from build123d import *

# Parameters (mm, degrees)
SKETCH1_W           = 200
SKETCH1_H           = 30
SKETCH1_W_2         = 20
SKETCH1_H_2         = 200
SKETCH1_R           = 4
BOSS_EXTRUDE1_DEPTH = 1


with BuildPart() as part:
    # Sketch1 → Boss-Extrude1 (new body)
    with BuildSketch(Plane.XY):
        with Locations((120, 100)):
            Rectangle(SKETCH1_W, SKETCH1_H)
        with Locations((10, 100)):
            Rectangle(SKETCH1_W_2, SKETCH1_H_2)
        with Locations((10, 175)):
            Circle(SKETCH1_R, mode=Mode.SUBTRACT)
        with Locations((10, 25)):
            Circle(SKETCH1_R, mode=Mode.SUBTRACT)
        Polygon((220, 200), (220, 115), (220, 85), (220, 0), (240, 0), (240, 200), align=None)
        with Locations((230, 25)):
            Circle(SKETCH1_R, mode=Mode.SUBTRACT)
        with Locations((230, 175)):
            Circle(SKETCH1_R, mode=Mode.SUBTRACT)
    extrude(amount=BOSS_EXTRUDE1_DEPTH)


solid = part.part
For this review, take the finished solid that the model builds, in its own axes (mm). Give positions to 0.01 mm unless a question says otherwise; leave off trailing zeros. Loops run counter-clockwise (first coordinate to the right, second up) from the corner with the lowest first, then second, coordinate; pieces in that order, holes last. Notation, with made-up numbers: M 3.5,22 L 48.5,22 A17 ccw 48.5,26 Z; hole C 85.25,32 d9. An arc over 180 degrees is marked long. Answer as a JSON object with one key per item and string values. Group by question number.
Q1. For probe 1 along Y at (x, z) = (230, 0.4); probe 2 along X at (y, z) = (174.5, 0.65); probe 3 along X at (y, z) = (192.5, 0.35), list the stretches that pass through material, from the lowest coordinate up. Write a range as [from, to].
Q2. Add section C-C on x = 230. Give the boundary of the cut face in (y, z).
Q3. Add section A-A on z = 0.45. Give the boundary of the cut face in (x, y).
Q4. Insertion check: P1, Ø13, axis at x = 230, y = 25, coming from the +Z side. The pin has a flat end and moves straight along its axis. Give the tip position at first contact, or say it passes through.
Q5. Add section D-D on y = 175. Give the boundary of the cut face in (x, z), and give its area (3 significant figures).
Q6. Add section B-B on y = 55.5. Give the boundary of the cut face in (x, z), and give its area (3 significant figures).
Q7. Mouldability with a two-part tool opening along Y and no side actions: class faces 1 (the cylindrical face through (227.05, 177.7, 0.49)), 2 (the flat face through (119, 108, 1)) as +Y half, -Y half, draft (parallel to the pull), parting line (faces both ways), or undercut.
Checked values:
{
 "1": {"probe 1": "[0, 21], [29, 171], [179, 200]", "probe 2": "[0, 6.03], [13.97, 20], [220, 226.03], [233.97, 240]", "probe 3": "[0, 20], [220, 240]"},
 "2": {"outline": "M 0,0 L 21,0 L 21,1 L 0,1 Z; M 29,0 L 171,0 L 171,1 L 29,1 Z; M 179,0 L 200,0 L 200,1 L 179,1 Z"},
 "3": {"outline": "M 0,0 L 20,0 L 20,85 L 220,85 L 220,0 L 240,0 L 240,200 L 220,200 L 220,115 L 20,115 L 20,200 L 0,200 Z; hole C 10,25 d8; hole C 10,175 d8; hole C 230,25 d8; hole C 230,175 d8"},
 "4": {"P1": "z = 1"},
 "5": {"outline": "M 0,0 L 6,0 L 6,1 L 0,1 Z; M 14,0 L 20,0 L 20,1 L 14,1 Z; M 220,0 L 226,0 L 226,1 L 220,1 Z; M 234,0 L 240,0 L 240,1 L 234,1 Z", "area": "24.0 mm²"},
 "6": {"outline": "M 0,0 L 20,0 L 20,1 L 0,1 Z; M 220,0 L 240,0 L 240,1 L 220,1 Z", "area": "40.0 mm²"},
 "7": {"face 1": "undercut", "face 2": "draft"}
}
